from build123d import *

# Parameters (mm, degrees)
BOSS_EXTRUDE1_DEPTH    = 66.04
SKETCH3_R              = 12.7
CUT_EXTRUDE1_DEPTH     = 2.1
SKETCH2_R              = 1.5
SKETCH2_R_2            = 3.81
CUT_EXTRUDE2_DEPTH     = 8
SKETCH4_R              = 2.2
BOSS_EXTRUDE2_DEPTH    = 20.32
SKETCH6_W              = 12.1468
SKETCH6_H              = 12
CUT_EXTRUDE3_DEPTH     = 4
SKETCH7_R              = 2.8
CUT_EXTRUDE4_DEPTH     = 1.27
SKETCH8_R              = 1.925
M4_BOTTOM_SCREWS_DEPTH = 4


with BuildPart() as part:
    # Sketch1 → Boss-Extrude1 (new body)
    with BuildSketch(Plane(origin=(0, 0, 0), x_dir=(0, 0, -1), z_dir=(1, 0, 0))):
        Polygon((7, 3), (27.32, 3), (27.32, 0), (2.660377358, 0), (0, 0), (0, 42.3), (7, 42.3), align=None)
    extrude(amount=BOSS_EXTRUDE1_DEPTH)

    # Sketch3 → Cut-Extrude1 (cut)
    with BuildSketch(Plane.XY):
        with Locations((21.15, 21.15)):
            Circle(SKETCH3_R)
    extrude(amount=-CUT_EXTRUDE1_DEPTH, mode=Mode.SUBTRACT)

    # Sketch2 → Cut-Extrude2 (cut, through all)
    with BuildSketch(Plane(origin=(0, 0, -7), x_dir=(-1, 0, 0), z_dir=(0, 0, -1))):
        with Locations((-5.65, 36.65)):
            Circle(SKETCH2_R)
        with Locations((-5.65, 5.65)):
            Circle(SKETCH2_R)
        with Locations((-36.65, 36.65)):
            Circle(SKETCH2_R)
        with Locations((-36.65, 5.65)):
            Circle(SKETCH2_R)
        with Locations((-21.15, 21.15)):
            Circle(SKETCH2_R_2)
    extrude(amount=-CUT_EXTRUDE2_DEPTH, mode=Mode.SUBTRACT)

    # Sketch4 → Boss-Extrude2 (add)
    with BuildSketch(Plane(origin=(0, 0, -7), x_dir=(-1, 0, 0), z_dir=(0, 0, -1))):
        with Locations((-49.852, 21.15)):
            Circle(SKETCH4_R)
    extrude(amount=BOSS_EXTRUDE2_DEPTH)

    # Sketch6 → Cut-Extrude3 (cut, through all)
    with BuildSketch(Plane(origin=(0, 3, 0), x_dir=(1, 0, 0), z_dir=(0, 1, 0))):
        with Locations((35.4276, 13)):
            Rectangle(SKETCH6_W, SKETCH6_H)
    extrude(amount=-CUT_EXTRUDE3_DEPTH, mode=Mode.SUBTRACT)

    # Sketch7 → Cut-Extrude4 (cut)
    with BuildSketch(Plane(origin=(0, 0, -7), x_dir=(-1, 0, 0), z_dir=(0, 0, -1))):
        with Locations((-36.65, 36.65)):
            Circle(SKETCH7_R)
        with Locations((-36.65, 5.65)):
            Circle(SKETCH7_R)
        with Locations((-5.65, 5.65)):
            Circle(SKETCH7_R)
        with Locations((-5.65, 36.65)):
            Circle(SKETCH7_R)
    extrude(amount=-CUT_EXTRUDE4_DEPTH, mode=Mode.SUBTRACT)

    # Sketch8 → M4 bottom screws (cut, through all)
    with BuildSketch(Plane(origin=(0, 3, 0), x_dir=(1, 0, 0), z_dir=(0, 1, 0))):
        with Locations((20.3542, 17.16)):
            Circle(SKETCH8_R)
        with Locations((53.501, 17.16)):
            Circle(SKETCH8_R)
    extrude(amount=-M4_BOTTOM_SCREWS_DEPTH, mode=Mode.SUBTRACT)


solid = part.part
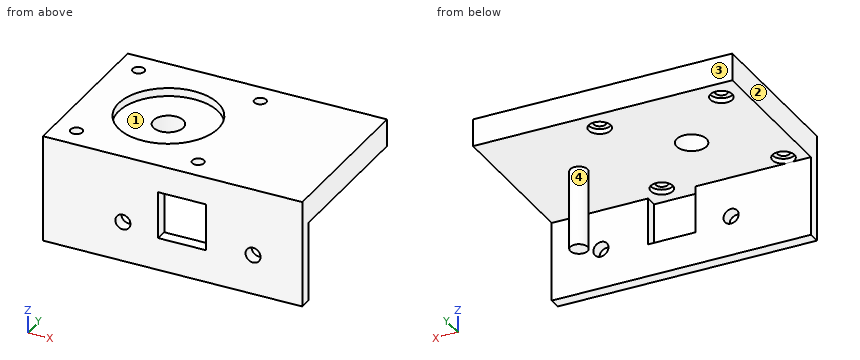
Source: CAD feature listing. Evaluate the final solid. Frame: model axes, mm. Face numbers are marked on the shaded views. Round coordinates to 2 decimals unless told otherwise and drop trailing zeros. Loops run counter-clockwise (first coordinate to the right, second up) from the corner with the lowest first, then second, coordinate; pieces in that order, holes last.
Q1. Mould query, pull axis Y, two halves, no side actions, for the marked faces 1, 2, 3 and 4. Classes: pulls with the +Y half, pulls with the -Y half, needs draft (parallel to the pull), parting line crosses it, or undercut.
Q2. Section D-D, the plane z = -17.16. Return loops of the section in (x, y), plus the area to 3 significant figures.
Q3. Section B-B, the plane z = -24.75. Return loops of the section in (x, y).
Q4. First-contact query: P1, Ø1.5, axis at x = 33, y = 2, coming from the +Z side; P2, Ø3, axis at x = 56.5, z = -17.5, coming from the +Y side; P3, Ø23, axis at x = 21.15, y = 21.15, coming from the -Z side; P4, Ø1.8, axis at x = 36.65, y = 5.65, coming from the +Z side. Flat tips, straight axial feed; report the tip coordinate or a pass-through.
Q5. Section C-C, the plane x = 36.65. Return loops of the section in (y, z).
Q6. Section A-A, the plane y = 21.15. Return loops of the section in (x, z).
Q7. Ray query, line 1 (Y direction, x = 5.65, z = -2.05); line 2 (X direction, y = 1.65, z = -17.16); line 3 (Y direction, x = 21.15, z = -0.5). Return the intervals inside material, ascending.
Solutions:
1. face 1: undercut
1. face 2: needs draft
1. face 3: pulls with the +Y half
1. face 4: undercut
2. outline: (0, 0) - (18.43, 0) - (18.43, 3) - (0, 3) - close; (22.28, 0) - (29.35, 0) - (29.35, 3) - (22.28, 3) - close; (41.5, 0) - (51.58, 0) - (51.58, 3) - (41.5, 3) - close; circle Ø4.4 at (49.85, 21.15); (55.43, 0) - (66.04, 0) - (66.04, 3) - (55.43, 3) - close
2. area: 154 mm2
3. outline: (0, 0) - (66.04, 0) - (66.04, 3) - (0, 3) - close; circle Ø4.4 at (49.85, 21.15)
4. P1: stops at z = 0
4. P2: stops at y = 3
4. P3: stops at z = -7
4. P4: passes through
5. outline: (0, -27.32) - (3, -27.32) - (3, -19) - (0, -19) - close; (0, -7) - (2.85, -7) - (2.85, -5.73) - (4.15, -5.73) - (4.15, 0) - (0, 0) - close; (7.15, -5.73) - (8.45, -5.73) - (8.45, -7) - (33.85, -7) - (33.85, -5.73) - (35.15, -5.73) - (35.15, 0) - (7.15, 0) - close; (38.15, -5.73) - (39.45, -5.73) - (39.45, -7) - (42.3, -7) - (42.3, 0) - (38.15, 0) - close
6. outline: (0, -7) - (17.34, -7) - (17.34, -2.1) - (8.45, -2.1) - (8.45, 0) - (0, 0) - close; (24.96, -7) - (47.65, -7) - (47.65, -27.32) - (52.05, -27.32) - (52.05, -7) - (66.04, -7) - (66.04, 0) - (33.85, 0) - (33.85, -2.1) - (24.96, -2.1) - close
7. line 1: y = 0 to 4.15, 7.15 to 35.15, 38.15 to 42.3
7. line 2: x = 0 to 18.43, 22.28 to 29.35, 41.5 to 51.58, 55.43 to 66.04
7. line 3: y = 0 to 8.45, 33.85 to 42.3
